For this review, take the finished solid that the model builds, in its own axes (mm). A direction names the side the tool comes from. Give positions to 0.01 mm unless a question says otherwise; leave off trailing zeros. Loops run counter-clockwise (first coordinate to the right, second up) from the corner with the lowest first, then second, coordinate; pieces in that order, holes last.
```python
from build123d import *

# Parameters (mm, degrees)
SKETCH1_W                    = 38.1
SKETCH1_H                    = 38.1
MAIN_BODY_DEPTH              = 34
F_9_32_RIGHT_RAIL_DEPTH      = 64.712008287
F_9_32_RIGHT_RAIL_DEPTH_BACK = 5.55625
SKETCH3_R                    = 3.571875
SKETCH4_R                    = 3.571875
F_9_32_LEFT_RAIL_DEPTH       = 5.55625
F_9_32_TOPPER_DEPTH          = 64.712008287
F_9_32_TOPPER_DEPTH_BACK     = 10
SKETCH8_R                    = 3.571875
HEX_START                    = -5.55625
HEX_HOLE_RIGHT_DEPTH         = 32.54375
HEX_HOLE_LEFT_DEPTH          = 32.54375
INNER_START                  = -34
INNER_CAVITY_OUTLINE_W       = 26.9875
INNER_CAVITY_OUTLINE_H       = 26.9875
INNER_CAVITY_DEPTH           = 25.26875
HEX_START_2                  = -17
HEX_HOLE_TOP_DEPTH           = 13.825
TOP_CORNER_REACH             = 65.712
SKETCH17_W                   = 1.5875
SKETCH17_H                   = 1.5875
CUT_EXTRUDE1_DEPTH           = 0.396875


# Read off the part's stored shape, not the designer's step: Inner Cavity
with BuildPart() as part:
    # Sketch1 → Main Body (new body)
    with BuildSketch(Plane(origin=(0, 0, 0), x_dir=(1, 0, 0), z_dir=(0, 1, 0))):
        with Locations((19.05, 19.05)):
            Rectangle(SKETCH1_W, SKETCH1_H)
    extrude(amount=MAIN_BODY_DEPTH)

    # Sketch3 → 9/32 Right Rail (cut, two sides: drawn at the far end of the back side and taken through both)
    with BuildSketch(Plane.XY.offset(-F_9_32_RIGHT_RAIL_DEPTH_BACK)):
        with Locations(Location((19.05, 17, 0), (0, 0, 180))):
            Circle(SKETCH3_R)
    extrude(amount=F_9_32_RIGHT_RAIL_DEPTH + F_9_32_RIGHT_RAIL_DEPTH_BACK, mode=Mode.SUBTRACT)

    # Sketch4 → 9/32 Left Rail (cut)
    with BuildSketch(Plane.ZY):
        with Locations((-19.05, 17)):
            Circle(SKETCH4_R)
    extrude(amount=-F_9_32_LEFT_RAIL_DEPTH, mode=Mode.SUBTRACT)

    # Sketch8 → 9/32 Topper (cut, two sides: drawn at the far end of the back side and taken through both)
    with BuildSketch(Plane(origin=(0, 34, 0), x_dir=(1, 0, 0), z_dir=(0, 1, 0)).offset(-F_9_32_TOPPER_DEPTH_BACK)):
        with Locations(Location((19.05, 19.05, 0), (0, 0, 90))):
            Circle(SKETCH8_R)
    extrude(amount=F_9_32_TOPPER_DEPTH + F_9_32_TOPPER_DEPTH_BACK, mode=Mode.SUBTRACT)

    # Sketch9 → Hex Hole Right (cut)
    with BuildSketch(Plane.ZY.offset(HEX_START)):
        Polygon((-22.315182739, 22.6554624), (-25.580365478, 17), (-22.315182739, 11.3445376), (-15.784817261, 11.3445376), (-12.519634522, 17), (-15.784817261, 22.6554624), align=None)
    extrude(amount=-HEX_HOLE_RIGHT_DEPTH, mode=Mode.SUBTRACT)

    # Sketch10 → Hex Hole Left (cut)
    with BuildSketch(Plane.XY.offset(HEX_START)):
        Polygon((15.784813595, 22.65546875), (12.51962719, 17), (15.784813595, 11.34453125), (22.315186405, 11.34453125), (25.58037281, 17), (22.315186405, 22.65546875), align=None)
    extrude(amount=-HEX_HOLE_LEFT_DEPTH, mode=Mode.SUBTRACT)

    # Inner Cavity outline → Inner Cavity (cut)
    with BuildSketch(Plane(origin=(0, 34, 0), x_dir=(1, 0, 0), z_dir=(0, 1, 0)).offset(INNER_START)):
        with Locations((24.60625, 24.60625)):
            Rectangle(INNER_CAVITY_OUTLINE_W, INNER_CAVITY_OUTLINE_H)
    extrude(amount=INNER_CAVITY_DEPTH, mode=Mode.SUBTRACT)

    # Sketch14 → Hex Hole Top (cut)
    with BuildSketch(Plane(origin=(0, 34, 0), x_dir=(1, 0, 0), z_dir=(0, 1, 0)).offset(HEX_START_2)):
        Polygon((24.70546875, 22.315186405), (19.05, 25.58037281), (13.39453125, 22.315186405), (13.39453125, 15.784813595), (19.05, 12.51962719), (24.70546875, 15.784813595), align=None)
    extrude(amount=HEX_HOLE_TOP_DEPTH, mode=Mode.SUBTRACT)

    # Sketch16 → Top Corner (cut, up to next)
    with BuildSketch(Plane(origin=(0, 34, 0), x_dir=(1, 0, 0), z_dir=(0, 1, 0)), mode=Mode.PRIVATE) as top_corner_sk1:
        Polygon((38.1, 38.1), (16.276714219, 38.1), (38.1, 16.276714219), align=None)
    top_corner_tool1 = extrude(top_corner_sk1.sketch, amount=-TOP_CORNER_REACH, mode=Mode.PRIVATE) & part.part
    add(top_corner_tool1.solids().sort_by_distance((30.825571, 34, -30.825571))[0], mode=Mode.SUBTRACT)

    # Sketch17 → Cut-Extrude1 (cut)
    with BuildSketch(Plane.XZ):
        with Locations((19.05, -5.55625)):
            Rectangle(SKETCH17_W, SKETCH17_H)
        with Locations((5.55625, -17.4625)):
            Rectangle(SKETCH17_W, SKETCH17_H)
        with Locations((5.55625, -20.6375)):
            Rectangle(SKETCH17_W, SKETCH17_H)
    extrude(amount=-CUT_EXTRUDE1_DEPTH, mode=Mode.SUBTRACT)


solid = part.part
```
Q1. Mouldability with a two-part tool opening along X and no side actions: class faces 1 (the flat face through (16.26, 28.01, -23.97)), 2 (the flat face through (8.295, 14.133, -14.175)), 3 (the flat face through (11.112, 12, -24)) as +X half, -X half, draft (parallel to the pull), parting line (faces both ways), or undercut.
Answers:
face 1: undercut
face 2: draft
face 3: +X half
Q2. Consider section D-D on y = 5.5. Give the boundary of the cut face in (x, z), plus the area to 3 significant figures.
Answers:
outline: (0, -38.1) - (11.11, -38.1) - (11.11, -11.11) - (38.1, -11.11) - (38.1, 0) - (0, 0) - close
area: 723 mm2
Q3. Consider section A-A on x = 7.5. Give the boundary of the cut face in (y, z).
Answers:
outline: (0, -38.1) - (34, -38.1) - (34, 0) - (0, 0) - close; hole (11.34, -22.32) - (17, -25.58) - (22.66, -22.32) - (22.66, -15.78) - (17, -12.52) - (11.34, -15.78) - close
Q4. For pin 1 Ø12 at (y, z) = (9, -25) entering from +X; pin 2 Ø5 at (x, y) = (27, 8.5) entering from -Z; pin 3 Ø13.5 at (x, z) = (29, -20.5) entering from -Y, all flat-tipped, find the tip position at first contact; note any pin that passes through.
Answers:
pin 1: stops at x = 11.11
pin 2: stops at z = -11.11
pin 3: stops at y = 25.27
Q5. For probe 1 along X at (y, z) = (17, -4.1); probe 2 along Y at (x, z) = (19.05, -3.9); probe 3 along Z at (x, y) = (7, 17), list the stretches that pass through material, from the lowest coordinate up.
Answers:
probe 1: x = 0 to 15.48, 22.62 to 38.1
probe 2: y = 0 to 13.43, 20.57 to 34
probe 3: z = -38.1 to -25.58, -12.52 to 0
Q6. Consider section B-B on z = -7.5. Give the boundary of the cut face in (x, y), plus the area to 3 significant figures.
Answers:
outline: (0, 0) - (38.1, 0) - (38.1, 34) - (0, 34) - close; hole (12.52, 17) - (15.78, 11.34) - (22.32, 11.34) - (25.58, 17) - (22.32, 22.66) - (15.78, 22.66) - close
area: 1,180 mm2
Q7. Consider section C-C on z = -19.05. Give the boundary of the cut face in (x, y) (1 decimal).
Answers:
outline: (0, 0) - (11.1, 0) - (11.1, 11.3) - (5.6, 11.3) - (5.6, 13.4) - (0, 13.4) - close; (0, 20.6) - (5.6, 20.6) - (5.6, 22.7) - (11.1, 22.7) - (11.1, 25.3) - (13.4, 25.3) - (13.4, 30.8) - (15.5, 30.8) - (15.5, 34) - (0, 34) - close; (22.6, 30.8) - (24.7, 30.8) - (24.7, 25.3) - (35.3, 25.3) - (35.3, 34) - (22.6, 34) - close
Q8. Machinability: for faces 4 (the flat face through (13.395, 28, -19)), 5 (the flat face through (5.556, 14.6, -16.2)), 6 (the cylindrical face through (2.739, 19.414, -21.683)), 7 (the flat face through (23.97, 19.79, -8.3)), which of the approach directions +Z, -Z, +X, -X, +Y, -Y give a long, thin tool a straight path to every point of the face, cutting with its end or side? Answer none if there is none.
Answers:
face 4: -Y
face 5: +X
face 6: +X, -X
face 7: -Z
